Could you check a few things on this model? Use its own coordinates, in mm. Round coordinates to 2 decimals unless told otherwise and drop trailing zeros. Loops run counter-clockwise (first coordinate to the right, second up) from the corner with the lowest first, then second, coordinate; pieces in that order, holes last. Notation, with made-up numbers: (89.5, 43) -> (103.5, 43) arc R18 ccw to (103.5, 61) -> close; hole circle Ø9 at (60.5, -9). An arc over 180 degrees is marked (long way). Put each result on its own line as item: value. Start each with the question number.
1. I'm going to push flat-ended pins straight in: P1, Ø22, axis at x = 0, y = 0, coming from the -Z side; P2, Ø6.5, axis at x = 0, y = 26, coming from the -Z side. Where does each tip first touch, or does it pass through?
2. Imagine slicing it at B-B, the plane z = 0.25. Please give me the cut outline in (x, y), and give its area (3 significant figures).
3. I need wall thicknesses on line 1 (Y direction, x = 0, z = 0.85); line 2 (Y direction, x = -2, z = 0.4); line 3 (Y direction, x = 27, z = 0.95). Which ranges of each line are inside material? Lowest first, please. Write a range as [from, to].
4. Imagine slicing it at C-C, the plane x = 9. Please give me the cut outline in (y, z), and give its area (3 significant figures).
5. Imagine slicing it at D-D, the plane y = -12. Please give me the cut outline in (x, z).
6. Imagine slicing it at A-A, the plane y = 0. Please give me the cut outline in (x, z).
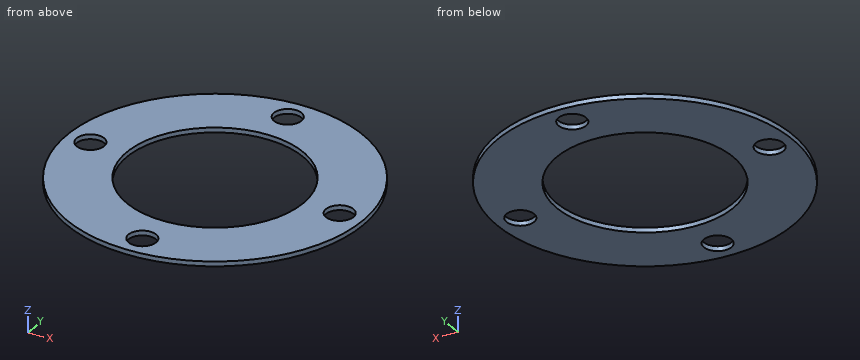
```python
from build123d import *

# Parameters (mm, degrees)
SKETCH1_R            = 31
SKETCH1_R_2          = 18.5
BOSS_EXTRUDE1_DEPTH  = 1
M5_CLEARANCE_HOLE1_D = 5.8


with BuildPart() as part:
    # Sketch1 → Boss-Extrude1 (new body)
    with BuildSketch(Plane.XY):
        Circle(SKETCH1_R)
        Circle(SKETCH1_R_2, mode=Mode.SUBTRACT)
    extrude(amount=BOSS_EXTRUDE1_DEPTH)

    # M5 Clearance Hole1 (through all)
    with Locations(Plane.XY.offset(1)):
        with Locations((26, 0), (0, 26), (-26, 0), (0, -26)):
            Hole(M5_CLEARANCE_HOLE1_D / 2)


solid = part.part
```
Entries:
1. P1: through
1. P2: z = 0
2. outline: circle Ø62 at (0, 0); hole circle Ø5.8 at (-26, 0); hole circle Ø37 at (0, 0); hole circle Ø5.8 at (0, -26); hole circle Ø5.8 at (0, 26); hole circle Ø5.8 at (26, 0)
2. area: 1,840 mm^2
3. line 1: [-31, -28.9], [-23.1, -18.5], [18.5, 23.1], [28.9, 31]
3. line 2: [-30.94, -28.1], [-23.9, -18.39], [18.39, 23.9], [28.1, 30.94]
3. line 3: [-15.23, -2.72], [2.72, 15.23]
4. outline: (-29.66, 0) -> (-16.16, 0) -> (-16.16, 1) -> (-29.66, 1) -> close; (16.16, 0) -> (29.66, 0) -> (29.66, 1) -> (16.16, 1) -> close
4. area: 27.0 mm^2
5. outline: (-28.58, 0) -> (-14.08, 0) -> (-14.08, 1) -> (-28.58, 1) -> close; (14.08, 0) -> (28.58, 0) -> (28.58, 1) -> (14.08, 1) -> close
6. outline: (-31, 0) -> (-28.9, 0) -> (-28.9, 1) -> (-31, 1) -> close; (-23.1, 0) -> (-18.5, 0) -> (-18.5, 1) -> (-23.1, 1) -> close; (18.5, 0) -> (23.1, 0) -> (23.1, 1) -> (18.5, 1) -> close; (28.9, 0) -> (31, 0) -> (31, 1) -> (28.9, 1) -> close
